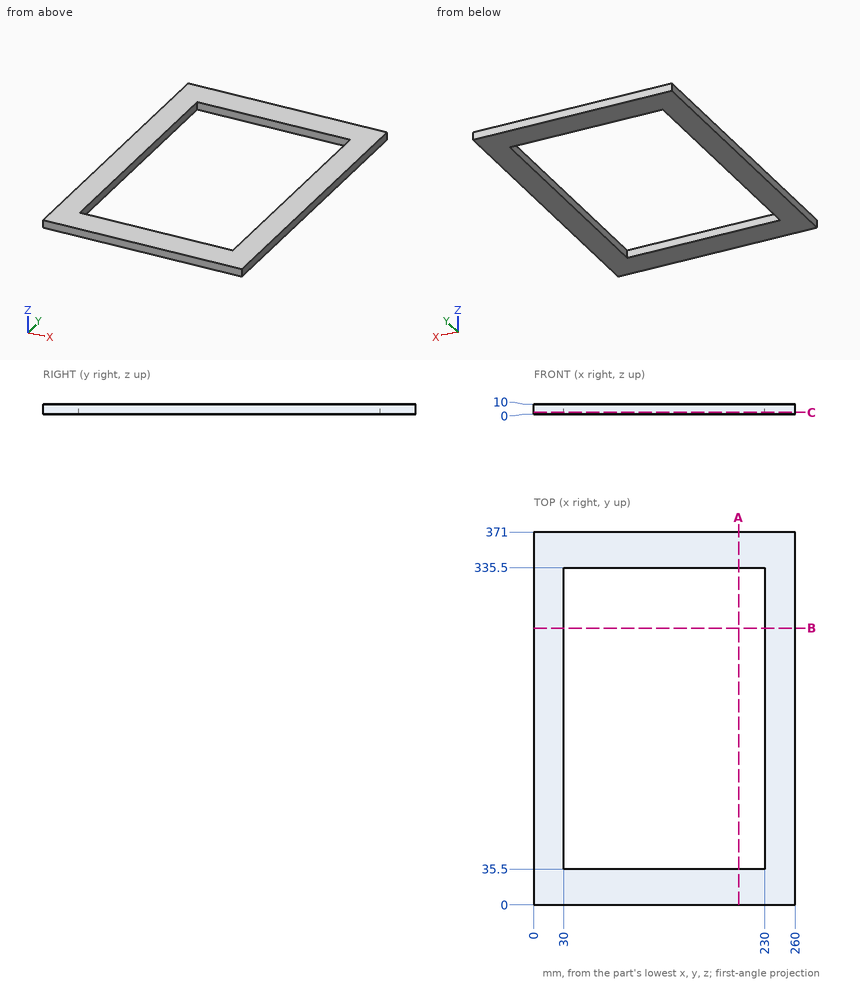
Study the drawing (mm; zero at the part's minimum x, y, z) and answer. Coordinates: 2 decimals unless noted, no trailing zeros. Order: outer loops, then holes, each group sorted by start corner. A loop starts at its lowest first (then second) coordinate and runs counter-clockwise, first axis right, second up. Notation, with made-up numbers: M 32.25,66 L 41.25,66 A14 cw 41.25,71 Z; hole C 7.5,31.5 d10. An arc over 180 degrees is marked long. Answer as a JSON object with one key per item and string values. Group by question number.
1. Section B-B on y = 275.5 is taken. Write down the section's boundary in (x, z), then the cut area to 3 significant figures.
2. Section C-C on z = 1.75 is taken. Write down the section's boundary in (x, y).
3. Section A-A on x = 204 is taken. Write down the section's boundary in (y, z).
4. A flat-ended cylindrical pin translates along its axis: P1, Ø2, axis at y = 327, z = 1, coming from the -X side. Find the tip coordinate at first contact, or state that the pin passes through.
5. Straight lines are drawn through the part: line 1 (Y direction, x = 163.5, z = 4); line 2 (X direction, y = 126, z = 8). For each, find the intervals that lie inside material, in ascending order.
Values follow:
{
 "1": {"outline": "M 0,0 L 30,0 L 30,10 L 0,10 Z; M 230,0 L 260,0 L 260,10 L 230,10 Z", "area": "600 mm2"},
 "2": {"outline": "M 0,0 L 260,0 L 260,371 L 0,371 Z; hole M 30,35.5 L 230,35.5 L 230,335.5 L 30,335.5 Z"},
 "3": {"outline": "M 0,0 L 35.5,0 L 35.5,10 L 0,10 Z; M 335.5,0 L 371,0 L 371,10 L 335.5,10 Z"},
 "4": {"P1": "x = 0"},
 "5": {"line 1": "0 to 35.5, 335.5 to 371", "line 2": "0 to 30, 230 to 260"}
}
